Check sheet for the modelled part. Datum: model origin and axes. Units: mm. A direction names the side the tool comes from. Give positions to 0.01 mm unless a question says otherwise; leave off trailing zeros. Write each loop counter-clockwise with the first axis right and the second up, starting at its lowest first coordinate (ties: lowest second). Pieces come first, ordered by that corner, then holes. Notation, with made-up numbers: (75, 52.25) -> (93, 52.25) arc R19 cw to (93, 79.25) -> close; hole circle Ø2 at (-35.5, 0). An arc over 180 degrees is marked (long way). Return JSON: item names as keys, results as strings.
from build123d import *

# Parameters (mm, degrees)
F1_DEPTH = 15
F0_R     = 2.7
F2_DEPTH = 5
F3_START = 10
F3_DEPTH = 5
F4_START = 5
F4_DEPTH = 5


with BuildPart() as f1:
    # F0 (on Top) → F1 (new body)
    with BuildSketch(Plane.XY):
        with BuildLine():
            ThreePointArc((128.9690721838, 41.7179030249), (59.4297181842, 16.601757413), (-13.5443023154, 4.7133236555))
            ThreePointArc((-13.5443023154, 4.7133236555), (-5.5454612916, -2.2522016138), (-12.5109865609, -10.2510426376))
            ThreePointArc((-12.5109865609, -10.2510426376), (63.1995597074, 2.0832073859), (135.346639482, 28.1412084582))
            ThreePointArc((135.346639482, 28.1412084582), (125.3695085496, 31.7407720924), (128.9690721838, 41.7179030249))
        make_face()
    extrude(amount=F1_DEPTH)

    # F0 (on Top) → F2 (join)
    with BuildSketch(Plane.XY):
        with BuildLine():
            ThreePointArc((-12.5109865609, -10.2510426376), (-5.5454612916, -2.2522016138), (-13.5443023154, 4.7133236555))
            ThreePointArc((-13.5443023154, 4.7133236555), (-20.5098275846, -3.2855173683), (-12.5109865609, -10.2510426376))
        make_face()
        with Locations((-13.0276444381, -2.768859491)):
            Circle(F0_R, mode=Mode.SUBTRACT)
    extrude(amount=F2_DEPTH)

    # F0 (on Top) → F3 (join)
    with BuildSketch(Plane.XY.offset(F3_START)):
        with BuildLine():
            ThreePointArc((-12.5109865609, -10.2510426376), (-5.5454612916, -2.2522016138), (-13.5443023154, 4.7133236555))
            ThreePointArc((-13.5443023154, 4.7133236555), (-20.5098275846, -3.2855173683), (-12.5109865609, -10.2510426376))
        make_face()
        with Locations((-13.0276444381, -2.768859491)):
            Circle(F0_R, mode=Mode.SUBTRACT)
    extrude(amount=F3_DEPTH)

    # F0 (on Top) → F4 (join)
    with BuildSketch(Plane.XY.offset(F4_START)):
        with BuildLine():
            ThreePointArc((135.346639482, 28.1412084582), (138.9462031162, 38.1183393907), (128.9690721838, 41.7179030249))
            ThreePointArc((128.9690721838, 41.7179030249), (125.3695085496, 31.7407720924), (135.346639482, 28.1412084582))
        make_face()
        with Locations((132.1578558329, 34.9295557416)):
            Circle(F0_R, mode=Mode.SUBTRACT)
    extrude(amount=F4_DEPTH)


solid = f1.part
(1) Depth check by flat-ended pin: pin 1 Ø8.5 at (x, y) = (132.16, 34.93) entering from -Z; pin 2 Ø4 at (x, z) = (104, 4.5) entering from -Y; pin 3 Ø1 at (y, z) = (-0.5, 8.5) entering from -X. Enter the tip coordinate at first touch or a pass-through.
Reply:
{"pin 1": "z = 5", "pin 2": "y = 14.22", "pin 3": "x = -6.06"}
(2) Thickness scan on L1, parallel to X at y = 33.5, z = 9.5; L2, parallel to Y at x = -4.5, z = 13.75; L3, parallel to Y at x = 110, z = 5. Record the ranges inside material, lowest first.
Reply:
{"L1": "110.25 to 129.87, 134.45 to 139.52", "L2": "-9.62 to 5.44", "L3": "17.25 to 33.4"}
(3) Release check for a two-part mould opening along Z. For faces 1 (the cylindrical face through (125.441, 31.592, 2.465)), 2 (the flat face through (57, 10, 0)), 3 (the cylindrical face through (-5.56, -2.09, 7.46)), 4 (the flat face through (-10, -3, 10)) record: pulls with the +Z half, pulls with the -Z half, needs draft (parallel to the pull), parting line crosses it, or undercut.
Reply:
{"face 1": "needs draft", "face 2": "pulls with the -Z half", "face 3": "undercut", "face 4": "undercut"}
(4) Set-up check for faces 5 (the flat face through (-10, -3, 5)), 6 (the cylindrical face through (125.441, 31.592, 12.465)), 7 (the cylindrical face through (-15.725, -2.65, 2.465)): record each of +Z, -Z, +X, -X, +Y, -Y from which the full face is reachable in a straight line by a thin tool's end or side.
Reply:
{"face 5": "-X", "face 6": "+Z", "face 7": "+Z, -Z"}
(5) Cross-section at D-D on y = 30. Enter the section's corners in (x, z).
Reply:
{"outline": "(101.38, 0) -> (126.51, 0) -> (126.51, 5) -> (137.81, 5) -> (137.81, 10) -> (126.51, 10) -> (126.51, 15) -> (101.38, 15) -> close"}
(6) Cross-section at A-A on z = 2.5. Enter the section's corners in (x, y).
Reply:
{"outline": "(-13.54, 4.71) arc R7.5 ccw to (-12.51, -10.25) arc R415 ccw to (135.35, 28.14) arc R7.5 cw to (128.97, 41.72) arc R400 cw to start; hole circle Ø5.4 at (-13.03, -2.77)"}
(7) Cross-section at B-B on y = 2.5. Enter the section's corners in (x, z).
Reply:
{"outline": "(-18.37, 0) -> (64.79, 0) -> (64.79, 15) -> (-18.37, 15) -> (-18.37, 10) -> (-7.69, 10) -> (-7.69, 5) -> (-18.37, 5) -> close"}
(8) Cross-section at C-C on x = 55. Enter the section's corners in (y, z), then the cut area to 3 significant figures.
Reply:
{"outline": "(0.04, 0) -> (15.48, 0) -> (15.48, 15) -> (0.04, 15) -> close", "area": "232 mm^2"}
